CAD build for the part. Positions are in the model's coordinates, mm. A direction names the side the tool comes from. Give positions to 0.01 mm unless a question says otherwise; leave off trailing zeros. Order: outer loops, then holes, each group sorted by start corner. A loop starts at its lowest first (then second) coordinate and runs counter-clockwise, first axis right, second up.
Item 1: Wall check: L1, parallel to Z at x = -10, y = 13.75; L2, parallel to Z at x = -12.75, y = 21; L3, parallel to X at y = 10.95, z = 65. Give the ranges that are in metal, low to high.
Item 2: Band-saw the part on C-C on y = 18.25. Give the cut face in (x, z), plus the area to 3 significant figures.
Item 3: Band-saw the part on B-B on x = -1.75. Give the cut face in (y, z).
Item 4: Which spindle directions (+Z, -Z, +X, -X, +Y, -Y) get a long thin tool onto all of the face, cutting with end or side? Do faces 1 (the flat face through (-10, 8, 0)), 2 (the flat face through (-10, 8, 60)), 3 (the flat face through (-12, 13, -3)), 4 (the flat face through (-2, 25, 10)), 5 (the flat face through (-12, 23, 60)). Say none if no direction does.
Item 5: Band-saw the part on D-D on z = 30. Give the cut face in (x, y).
Item 6: Flat gauge pins, fed straight in: P1, Ø9, axis at x = -9.97, z = -5, coming from the -Y side; P2, Ø2.5, axis at x = -3, y = 23, coming from the +Z side; P3, Ø5, axis at x = -7.5, z = 64.5, coming from the +Y side. Where does each tip first touch, or does it go through?
Item 7: Band-saw the part on A-A on z = 65. Give the cut face in (x, y).
```python
from build123d import *

# Parameters (mm, degrees)
BOSS_EXTRU_1_DEPTH                                = 60
ENL_V_MAT_EXTRU_1_DEPTH                           = 20
ENL_V_MAT_EXTRU_2_DEPTH                           = 56
ENL_V_MAT_EXTRU_2_DEPTH_BACK                      = 6
BOSS_EXTRU_2_DEPTH                                = 10
CHAMBRAGE_POUR_VIS_SIX_PANS_CREUX_M41_D           = 4.8
CHAMBRAGE_POUR_VIS_SIX_PANS_CREUX_M41_CBORE_D     = 8
CHAMBRAGE_POUR_VIS_SIX_PANS_CREUX_M41_CBORE_DEPTH = 2


with BuildPart() as part:
    # Esquisse1 → Boss.-Extru.1 (new body)
    with BuildSketch(Plane.XY):
        with BuildLine():
            Line((-19.942668722, 35), (-19.942668722, 10))
            Line((-19.942668722, 10), (-12.342668722, 10))
            Line((-12.342668722, 10), (-12.342668722, 8))
            ThreePointArc((-12.342668722, 8), (-9.942668722, 5.6), (-7.542668722, 8))
            Line((-7.542668722, 8), (-7.542668722, 10))
            Line((-7.542668722, 10), (0.057331278, 10))
            Line((0.057331278, 10), (0.057331278, 35))
            Line((0.057331278, 35), (-19.942668722, 35))
        make_face()
    extrude(amount=BOSS_EXTRU_1_DEPTH)

    # Esquisse2 → Enlèv. mat.-Extru.1 (cut)
    with BuildSketch(Plane(origin=(0, 35, 0), x_dir=(1, 0, 0), z_dir=(0, 1, 0))):
        Polygon((0.057331278, -50), (0.057331278, -10), (-4.942668722, -10), (-4.942668722, -5), (-14.942668722, -5), (-14.942668722, -55), (-4.942668722, -55), (-4.942668722, -50), align=None)
    extrude(amount=-ENL_V_MAT_EXTRU_1_DEPTH, mode=Mode.SUBTRACT)

    # Esquisse3 → Enlèv. mat.-Extru.2 (cut, two sides)
    with BuildSketch(Plane.XY.offset(5)) as enl_v_mat_extru_2_sk:
        with BuildLine():
            ThreePointArc((-8.824634733, 27.236067977), (-12.178736699, 26.118033989), (-11.06070271, 22.763932023))
            Line((-11.06070271, 22.763932023), (-8.824634733, 27.236067977))
        make_face()
        with BuildLine():
            Line((-8.824634733, 27.236067977), (-11.06070271, 22.763932023))
            ThreePointArc((-11.06070271, 22.763932023), (-8.628340941, 22.873372979), (-7.442668722, 25))
            ThreePointArc((-7.442668722, 25), (-7.816041701, 26.31432778), (-8.824634733, 27.236067977))
        make_face()
    extrude(amount=ENL_V_MAT_EXTRU_2_DEPTH, mode=Mode.SUBTRACT)
    extrude(enl_v_mat_extru_2_sk.sketch, amount=-ENL_V_MAT_EXTRU_2_DEPTH_BACK, mode=Mode.SUBTRACT)

    # Esquisse4 → Boss.-Extru.2 (add)
    with BuildSketch(Plane.XY.offset(60)):
        Polygon((-19.942668722, 15), (-19.942668722, 10), (-12.342668722, 10), (-7.542668722, 10), (0.057331278, 10), (0.057331278, 15), align=None)
    boss_extru_2 = extrude(amount=BOSS_EXTRU_2_DEPTH)

    # Symétrie1: Boss.-Extru.2 across plane
    add(boss_extru_2.mirror(Plane.XY.offset(30)))

    # Chambrage pour vis à six pans creux M41 (through all)
    with Locations(Plane(origin=(-9.971334361, 15, -5), x_dir=(0, 0, 1), z_dir=(0, 1, 0))):
        with Locations((0, 0), (70, 0.028665639)):
            CounterBoreHole(CHAMBRAGE_POUR_VIS_SIX_PANS_CREUX_M41_D / 2, CHAMBRAGE_POUR_VIS_SIX_PANS_CREUX_M41_CBORE_D / 2, CHAMBRAGE_POUR_VIS_SIX_PANS_CREUX_M41_CBORE_DEPTH)


solid = part.part
```
The answers:
1. L1: z = -10 to -9, -1 to 61, 69 to 70
1. L2: z = 0 to 5, 55 to 60
1. L3: x = -19.94 to -12.34, -7.54 to 0.06
2. outline: (-19.94, 0) - (0.06, 0) - (0.06, 10) - (-4.94, 10) - (-4.94, 5) - (-14.94, 5) - (-14.94, 55) - (-4.94, 55) - (-4.94, 50) - (0.06, 50) - (0.06, 60) - (-19.94, 60) - close
2. area: 500 mm2
3. outline: (10, -10) - (15, -10) - (15, 0) - (35, 0) - (35, 10) - (15, 10) - (15, 50) - (35, 50) - (35, 60) - (15, 60) - (15, 70) - (10, 70) - close
4. face 1: -Z, +X, -X, -Y
4. face 2: +Z, +X, -X, -Y
4. face 3: +Y
4. face 4: +X, +Y
4. face 5: +Z, +X, -X, +Y
5. outline: (-19.94, 10) - (-12.34, 10) - (-12.34, 8) arc R2.4 ccw to (-7.54, 8) - (-7.54, 10) - (0.06, 10) - (0.06, 15) - (-14.94, 15) - (-14.94, 35) - (-19.94, 35) - close
6. P1: stops at y = 10
6. P2: stops at z = 60
6. P3: stops at y = 15
7. outline: (-19.94, 10) - (-12.34, 10) - (-12.34, 13) - (-13.94, 13) - (-13.94, 15) - (-19.94, 15) - close; (-7.54, 10) - (0.06, 10) - (0.06, 15) - (-5.94, 15) - (-5.94, 13) - (-7.54, 13) - close
